Source: CAD feature listing. Evaluate the final solid. Frame: model axes, mm. A direction names the side the tool comes from. Give positions to 0.01 mm unless a question says otherwise; leave off trailing zeros. Loops run counter-clockwise (first coordinate to the right, second up) from the corner with the lowest first, then second, coordinate; pieces in that order, holes last. Notation, with made-up numbers: (-27, -18) -> (-19, -18) arc R19 cw to (-19, 2) -> close; hole circle Ø5 at (75, 74). An arc over 180 degrees is marked (long way). Answer as a JSON object with one key per item and string values. Group by question number.
from build123d import *

# Parameters (mm, degrees)
F0_W     = 300
F0_H     = 350
F1_DEPTH = 125
F2_T     = -2.5
F3_R     = 5
F4_W     = 276.946939528
F4_H     = 325.1978382468
F5_DEPTH = 120


with BuildPart() as f1:
    # F0 (on Front) → F1 (new body)
    with BuildSketch(Plane.XZ):
        with Locations((95.7486510277, 99.5076403022)):
            Rectangle(F0_W, F0_H)
    extrude(amount=-F1_DEPTH)

    # F2 (hollow: no face is removed)
    offset(amount=F2_T, mode=Mode.SUBTRACT)

    # F3
    f3_edges = [f1.edges().sort_by_distance(p)[0] for p in [
        (245.748651, 62.5, 274.50764),
        (95.748651, 125, 274.50764),
        (245.748651, 125, 99.50764),
        (-54.251349, 125, 99.50764),
        (-54.251349, 62.5, 274.50764),
        (95.748651, 0, 274.50764),
        (245.748651, 0, 99.50764),
        (-54.251349, 0, 99.50764),
    ]]
    fillet(f3_edges, radius=F3_R)

    # F4 (on face) → F5 (cut)
    with BuildSketch(Plane(origin=(0, 125, 0), x_dir=(-1, 0, 0), z_dir=(0, 1, 0))):
        with Locations((-94.6279279888, 98.5161848366)):
            Rectangle(F4_W, F4_H)
    extrude(amount=-F5_DEPTH, mode=Mode.SUBTRACT)


solid = f1.part
(1) First-contact query: pin 1 (0.8 mm diameter, centred on y = 124, z = 117.5, fed in from +X); pin 2 (0.8 mm diameter, centred on x = 108, y = 123.5, fed in from +Z); pin 3 (0.8 mm diameter, centred on y = 124, z = 79, fed in from -X). Flat tips, straight axial feed; report the tip coordinate or a pass-through.
(2) Section query C-C on x = -25.5. Return the cut outline in (y, z).
(3) Material intervals for line 1 (X direction, y = 119, z = 225.5); line 2 (Z direction, x = 176.5, y = 108); line 3 (Y direction, x = 168, z = 220), sorted ascending. Write a range as from..to.
(4) Access query for faces 5 (the face through (-51.751, 62, 97)), 6 (the face through (94, 0, 99)). Directions: +Z, -Z, +X, -X, +Y, -Y. A direction counts if a zero-diameter tool reaches every point of the face in a straight line with its end or side. Return the directions, or none.
(5) Section query A-A on y = 58.5. Return the cut outline in (x, z).
(6) Section query B-B on z = 111. Return the cut outline in (x, y), plus the area to 3 significant figures.
(7) Mould query, pull axis Z, two halves, no side actions, for faces 1 (the face through (94, 62, 272.008)), 2 (the face through (-47, 122.5, 100)), 3 (the face through (94, 62, 274.508)), 4 (the face through (245.749, 62, 95)). Classes: pulls with the +Z half, pulls with the -Z half, needs draft (parallel to the pull), parting line crosses it, or undercut.
Result:
{
 "1": {"pin 1": "x = 244.22", "pin 2": "z = 273.43", "pin 3": "x = -52.72"},
 "2": {"outline": "(0, -75.49) -> (125, -75.49) -> (125, -64.08) -> (122.5, -64.08) -> (122.5, -72.99) -> (2.5, -72.99) -> (2.5, 272.01) -> (122.5, 272.01) -> (122.5, 261.12) -> (125, 261.12) -> (125, 269.51) arc R5 ccw to (120, 274.51) -> (5, 274.51) arc R5 ccw to (0, 269.51) -> close"},
 "3": {"line 1": "-54.25..-51.75, 243.25..245.75", "line 2": "-75.49..-72.99, 272.01..274.51", "line 3": "0..2.5"},
 "4": {"face 5": "none", "face 6": "+Z, -Z, +X, -X, -Y"},
 "5": {"outline": "(-54.25, -75.49) -> (245.75, -75.49) -> (245.75, 269.51) arc R5 ccw to (240.75, 274.51) -> (-49.25, 274.51) arc R5 ccw to (-54.25, 269.51) -> close; hole (-51.75, -72.99) -> (243.25, -72.99) -> (243.25, 272.01) -> (-51.75, 272.01) -> close"},
 "6": {"outline": "(-54.25, 5) arc R5 ccw to (-49.25, 0) -> (240.75, 0) arc R5 ccw to (245.75, 5) -> (245.75, 120) arc R5 ccw to (240.75, 125) -> (233.1, 125) -> (233.1, 122.5) -> (243.25, 122.5) -> (243.25, 2.5) -> (-51.75, 2.5) -> (-51.75, 122.5) -> (-43.85, 122.5) -> (-43.85, 125) -> (-49.25, 125) arc R5 ccw to (-54.25, 120) -> close", "area": "1,390 mm²"},
 "7": {"face 1": "undercut", "face 2": "undercut", "face 3": "pulls with the +Z half", "face 4": "needs draft"}
}
